from build123d import *

# Parameters (mm, degrees)
SKETCH_R             = 35
SKETCH_R_2           = 15
PAD_DEPTH            = 3
POCKET_DEPTH         = 198.081792
POCKET_DEPTH_BACK    = 201.081792
POLARPATTERN_COUNT   = 18
SKETCH002_R          = 19
SKETCH002_R_2        = 17.56
PAD001_DEPTH         = 20
SKETCH003_R          = 1.5
POCKET001_DEPTH      = 35.001
POCKET001_DEPTH_BACK = 35.001


with BuildPart() as part:
    # Sketch → Pad (new body)
    with BuildSketch(Plane.XY):
        Circle(SKETCH_R)
        Circle(SKETCH_R_2, mode=Mode.SUBTRACT)
    extrude(amount=PAD_DEPTH)

    # Sketch001 → Pocket (cut, two sides)
    with BuildSketch(Plane.XY) as pocket_sk:
        with BuildLine():
            ThreePointArc((25.8, 2), (23.8, 0), (25.8, -2))
            Line((25.8, -2), (30.6, -2))
            ThreePointArc((30.6, -2), (32.6, 0), (30.6, 2))
            Line((25.8, 2), (30.6, 2))
        make_face()
    pocket = extrude(amount=-POCKET_DEPTH, mode=Mode.SUBTRACT) + extrude(pocket_sk.sketch, amount=POCKET_DEPTH_BACK, mode=Mode.SUBTRACT)

    # PolarPattern: Pocket ×18 about axis
    polarpattern_axis = Axis((0, 0, 0), (0, 0, 1))
    for i in range(1, POLARPATTERN_COUNT):
        add(pocket.rotate(polarpattern_axis, i * 360 / POLARPATTERN_COUNT), mode=Mode.SUBTRACT)

    # Sketch002 → Pad001 (join)
    with BuildSketch(Plane.XY):
        Circle(SKETCH002_R)
        Circle(SKETCH002_R_2, mode=Mode.SUBTRACT)
    extrude(amount=PAD001_DEPTH)

    # Sketch003 → Pocket001 (cut, two sides)
    with BuildSketch(Plane.YZ) as pocket001_sk:
        with Locations((0, 5)):
            Circle(SKETCH003_R)
    extrude(amount=-POCKET001_DEPTH, mode=Mode.SUBTRACT)
    extrude(pocket001_sk.sketch, amount=POCKET001_DEPTH_BACK, mode=Mode.SUBTRACT)


solid = part.part
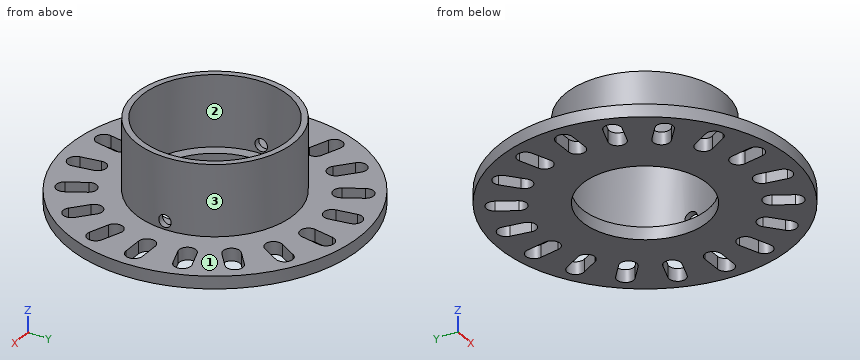
Can you work these out from the model? Positions are in its coordinate system, mm. Face numbers are marked on the shaded views. Round coordinates to 2 decimals unless told otherwise and drop trailing zeros. Loops run counter-clockwise (first coordinate to the right, second up) from the corner with the lowest first, then second, coordinate; pieces in that order, holes last. Notation, with made-up numbers: (86.25, 39) - (113.25, 39) arc R24 ccw to (113.25, 75) - close; hole circle Ø9 at (54, 5). An arc over 180 degrees is marked (long way). Use CSV: the item, a comma, the result in double quotes. Start each with the question number.
1) If we section it at C-C on y = 22.5: Write out the boundary of the cut face in (x, z), plus the area to 3 significant figures.
2) We'd pull the mould along Y, two halves only. Please class the marked faces 1, 2 and 3: released by +Y, released by -Y, zero draft, split by the parting line, or undercut.
3) For pin 1 Ø0.9 at (x, z) = (29, 2) entering from -Y; pin 2 Ø2.5 at (x, z) = (-28, 1.5) entering from -Y; pin 3 Ø2.5 at (x, z) = (28, 2) entering from +Y, each with a flat end and sliding along its axis, tell me the tip position at first contact or that it passes through.
4) If we section it at A-A on y = 0: Count the separate pieces of the cut face and the enclosed holes in it, plus the area to 3 significant figures.
5) If we section it at D-D on x = -8.5: Write out the boundary of the cut face in (y, z), plus the area to 3 significant figures.
6) Please list where these lines run through material, in increasing order: probe 1 along Z at (x, y) = (18, 0); probe 2 along X at (y, z) = (0, 14.5); probe 3 along X at (y, z) = (21.5, 2). Write a range as [from, to].
Geometry results:
1,outline,"(-26.81, 0) - (-15.3, 0) - (-15.3, 3) - (-26.81, 3) - close; (-10.91, 0) - (10.91, 0) - (10.91, 3) - (-10.91, 3) - close; (15.3, 0) - (26.81, 0) - (26.81, 3) - (15.3, 3) - close"
1,area,"134 mm2"
2,face 1,"zero draft"
2,face 2,"undercut"
2,face 3,"split by the parting line"
3,pin 1,"stops at y = -20.25"
3,pin 2,"stops at y = -22.57"
3,pin 3,"stops at y = 22.57"
4,separate pieces,"6"
4,enclosed holes,"0"
4,area,"108 mm2"
5,outline,"(-33.95, 0) - (-12.36, 0) - (-12.36, 3) - (-15.37, 3) - (-15.37, 20) - (-16.99, 20) - (-16.99, 3) - (-33.95, 3) - close; (12.36, 0) - (33.95, 0) - (33.95, 3) - (16.99, 3) - (16.99, 20) - (15.37, 20) - (15.37, 3) - (12.36, 3) - close"
5,area,"185 mm2"
6,probe 1,"z = [0, 3.5], [6.5, 20]"
6,probe 2,"x = [-19, -17.56], [17.56, 19]"
6,probe 3,"x = [-27.62, -24.25], [-22.64, -14.72], [-11.09, 11.09], [14.72, 22.64], [24.25, 27.62]"
